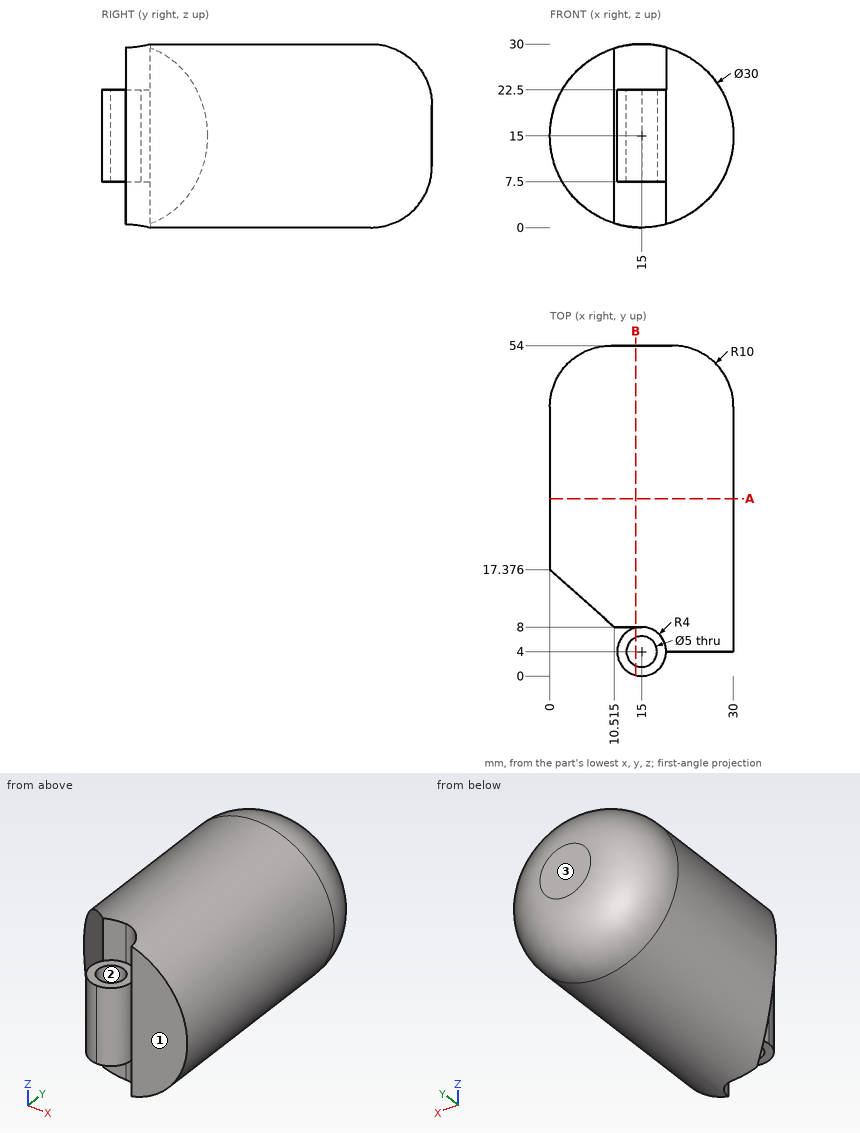
The drawing under review shows one solid part. Ordinate dimensions are in mm from its lowest x, y, z. Round coordinates to 2 decimals unless told otherwise and drop trailing zeros. Order: outer loops, then holes, each group sorted by start corner. A loop starts at its lowest first (then second) coordinate and runs counter-clockwise, first axis right, second up. Notation, with made-up numbers: (-1, 29) -> (29, 29) arc R37 ccw to (29, 68) -> close; hole circle Ø1 at (-26, 18.5). An arc over 180 degrees is marked (long way). Use a Markdown table: item, result.
Q1. For line 1 (X direction, y = 31, z = 19.5); line 2 (Z direction, x = 18.5, y = 45.5); line 3 (Z direction, x = 14.5, y = 9.5), list the stretches that pass through material, from the lowest coordinate up.
Values:
| item | result |
|---|---|
| line 1 | x = 0.69 to 29.31 |
| line 2 | z = 0.53 to 29.47 |
| line 3 | z = 0.01 to 29.99 |
Q2. We need section B-B on x = 14. State how many separate pieces and enclosed holes the cut face has, then the cut area to 3 significant figures.
Values:
| item | result |
|---|---|
| separate pieces | 3 |
| enclosed holes | 0 |
| area | 1,380 mm^2 |
Q3. Clearance check with flat-ended pins moving along their axes: P1, Ø1, axis at x = 17, z = 7.5, coming from the -Y side; P2, Ø8, axis at x = 8.5, z = 8.5, coming from the -Y side; P3, Ø6.5, axis at x = 15, y = 4, coming from the +Z side. State where each tip first meets the part, or that it passes through.
Values:
| item | result |
|---|---|
| P1 | stops at y = 0.29 |
| P2 | stops at y = 0.88 |
| P3 | stops at z = 22.5 |
Q4. We need section A-A on y = 29. Write out the cut boundary in (x, z), then the cut area to 3 significant figures.
Values:
| item | result |
|---|---|
| outline | circle Ø30 at (15, 15) |
| area | 707 mm^2 |
Q5. Mouldability with a two-part tool opening along Y and no side actions: class the marked faces 1, 2 and 3 as +Y half, -Y half, draft (parallel to the pull), parting line (faces both ways), or undercut.
Values:
| item | result |
|---|---|
| face 1 | -Y half |
| face 2 | undercut |
| face 3 | +Y half |
